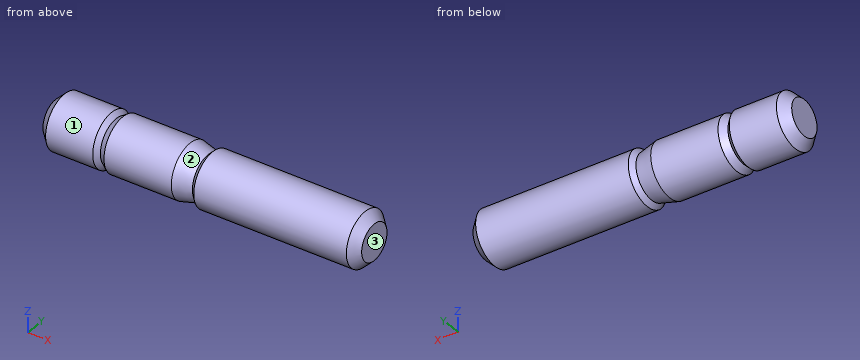
Autodesk Inventor part; units mm, degrees
ref_plane "Work Plane1" through (2.75, 0, 0) normal (0, -1, 0) x (1, 0, 0)
ref_plane "YZ Plane" through (0, 0, 0) normal (1, 0, 0) x (0, 1, 0)
ref_plane "XZ Plane" through (0, 0, 0) normal (0, 1, 0) x (-1, 0, 0)
sketch "Szkic1" plane through (0, 0, 0) normal (0, 0, 1) x (1, 0, 0)
  line L0 (28, 3) -> (28, 0)
  line L1 (-7.5, 0) -> (28, 0)
  line L2 (-14.6, 0) -> (35.1, 0)
  line L3 (0, 3.6) -> (0, -0.6)
  line L4 (-7.5, 3) -> (-7.5, 0)
  line L5 (10, 3) -> (10, 0) construction
  line L6 (-14.6, 0) -> (35.1, 0)
  line L7 (-7.5, 3) -> (28, 3)
  dimension "d4" = 7.5
  dimension "d5" = 28
  dimension "d6" = 18
  dimension "d13" = 6
revolve "Bryła" add sketch "Szkic1" angle 360 about axis through (-7.5, 0, 0) along (1, 0, 0)
thread "Gwint1"
thread "Gwint2"
chamfer "Faza1" distance 1 angle 45 1 edges at (-7.5, -3, 0) measured on face at (16.1667, 2.9903, -0.2414)
chamfer "Faza2" distance 1 angle 45 1 edges at (28, -3, 0) measured on face at (16.5, 2.9903, -0.2414)
sketch "Sketch5" plane through (0, 0, 0) normal (0, 0, 1) x (1, 0, 0)
  line L0 (-6.5, 3) -> (27, 3)
  line L1 (-6.5, -3) -> (27, -3)
  line L2 (28, 2) -> (28, -2)
  line L3 (-7.5, -2) -> (-7.5, 2)
  line L4 (10, 3) -> (9.5, 2.5)
  line L5 (9.5, 2.5) -> (7.5, 3)
  line L6 (-14.6, 0) -> (35.1, 0)
  point P0 (0, 0)
  dimension "d87" = 45
  dimension "d90" = 18
  dimension "d91" = 0.5
  dimension "d92" = 2.5
revolve "IDS_REVOLUTION{1}" cut sketch "Sketch5" angle 360 about axis through (-10, 0, 0) along (1, 0, 0)
sketch "Sketch6" plane through (0, 0, 0) normal (0, 0, 1) x (1, 0, 0)
  line L0 (-6.5, 3) -> (7.5, 3)
  line L1 (-7.5, -2) -> (-7.5, 2)
  line L2 (-1.25, 3) -> (-0.75, 2.5)
  line L3 (-0.75, 2.5) -> (0, 3)
  line L4 (-10.5, 0) -> (10.5, 0)
  point P0 (0, 0)
  dimension "d94" = 45
  dimension "d95" = 7.5
  dimension "d96" = 0.5
  dimension "d97" = 1.25
revolve "IDS_REVOLUTION{2}" cut sketch "Sketch6" angle 360 about axis through (-10, 0, 0) along (1, 0, 0)
ref_plane "Work Plane1" through (2.75, 0, 0) normal (0, -1, 0) x (1, 0, 0)
equation "\"d4\" = KOH"
equation "\"d5\" = NLG"
equation "\"d6\" = GEL"
equation "\"d13\" = GD"
equation "\"d1\" = KOH"
equation "\"d7\" = GEL"
equation "\"d9\" = -0.5 * SPD + 0.5 * GD"
equation "\"d10\" = -0.5 * SPD + 0.5 * GD"
equation "\"d11\" = -0.5 * SPD + 0.5 * GD"
equation "\"d12\" = -0.5 * SPD + 0.5 * GD"
equation "\"d90\" = GEL"
equation "\"d91\" = -0.25 * SPD + 0.25 * GD"
equation "\"d92\" = X1"
equation "\"d95\" = KOH"
equation "\"d96\" = -0.25 * SPD + 0.25 * GD"
equation "\"d97\" = X2"
equation "\"NLG\" = 28"
equation "\"GEL\" = 18"
equation "\"GAL\" = 0.61345 * PTC"
equation "\"SPD\" = 4"
equation "\"d0\" = GD"
equation "\"GUL\" = 0.61345 * PTC"
equation "\"KOH\" = 7.5"
equation "\"GD\" = 6"
equation "\"BDM\" = NND"
equation "\"GUL1\" = GUL"
equation "\"GAL1\" = GAL"
equation "\"d80\" = -GUL - GEL"
equation "\"d86\" = -KOH + GUL1"
equation "\"X1\" = 2.5"
equation "\"X2\" = 1.25"
equation "\"PTC\" = 1"
equation "\"THREADDIA\" = 6"
equation "\"TOA\" = 30deg"
equation "\"NND\" = 6"
equation "\"GD1\" = THREADDIA - 1.2269 * PTC"
properties part number "DIN 939 - M6 x 28" material "Stal, miękka"
Source: CAD feature listing. Evaluate the final solid. Frame: model axes, mm. Face numbers are marked on the shaded views. Coordinates: 2 decimals unless noted, no trailing zeros. Order: outer loops, then holes, each group sorted by start corner. A loop starts at its lowest first (then second) coordinate and runs counter-clockwise, first axis right, second up. Notation, with made-up numbers: M 48,44 L 94,44 A22 ccw 94,58 Z; hole C 42,-18.75 d1. An arc over 180 degrees is marked long. Write each question's results on one line, items separated by ' | '. Start each with the question number.
1. Section A-A, the plane z = 0. Return the cut outline in (x, y).
2. Material intervals for L1, parallel to Z at x = -6, y = 0.15; L2, parallel to Y at x = 17.5, z = 1.35, sorted ascending.
3. Draft query along X for the marked faces 1, 2 and 3. Return one class per face: +X half, -X half, draft (parallel to the pull), parting line (faces both ways), or undercut.
4. Section C-C, the plane x = 17. Return the cut outline in (y, z).
Solution:
1) outline: M -7.5,-2 L -6.5,-3 L -1.25,-3 L -0.75,-2.5 L 0,-3 L 7.5,-3 L 9.5,-2.5 L 10,-3 L 27,-3 L 28,-2 L 28,2 L 27,3 L 10,3 L 9.5,2.5 L 7.5,3 L 0,3 L -0.75,2.5 L -1.25,3 L -6.5,3 L -7.5,2 Z
2) L1: -3 to 3 | L2: -2.68 to 2.68
3) face 1: draft | face 2: undercut | face 3: +X half
4) outline: C 0,0 d6
